Can you work these out from the drawing? Everything is in mm from the part's minimum corner. Coordinates: 2 decimals unless noted, no trailing zeros. Order: outer loops, then holes, each group sorted by start corner. A loop starts at its lowest first (then second) coordinate and runs counter-clockwise, first axis right, second up. Notation, with made-up numbers: (47, 2) - (89, 2) arc R7 cw to (89, 11) - close; hole circle Ø1 at (-25.75, 88.25). An arc over 180 degrees is marked (long way). Use a Markdown table: item, result. Add a question column.
(1) I want a section at C-C (y = 1.5). List the corners of the cut face in (x, z) for me.
(2) I want a section at A-A (y = 4.75). List the corners of the cut face in (x, z) for me (1 decimal).
(3) I want a section at B-B (z = 1). List the corners of the cut face in (x, y) for me (1 decimal).
(4) If I drill on L1, parallel to X at y = 1.25, z = 0.5; L2, parallel to X at y = 6.75, z = 0.35 (1 decimal); L3, parallel to Y at x = 19, z = 0.2 (1 decimal), over which ranges is the centre line in solid material (lowest first)? Write a range as [from, to].
(5) We'd pull the mould along X, two halves only. Please class the marked faces 1 and 2: pulls with the +X half, pulls with the -X half, needs draft (parallel to the pull), parting line crosses it, or undercut.
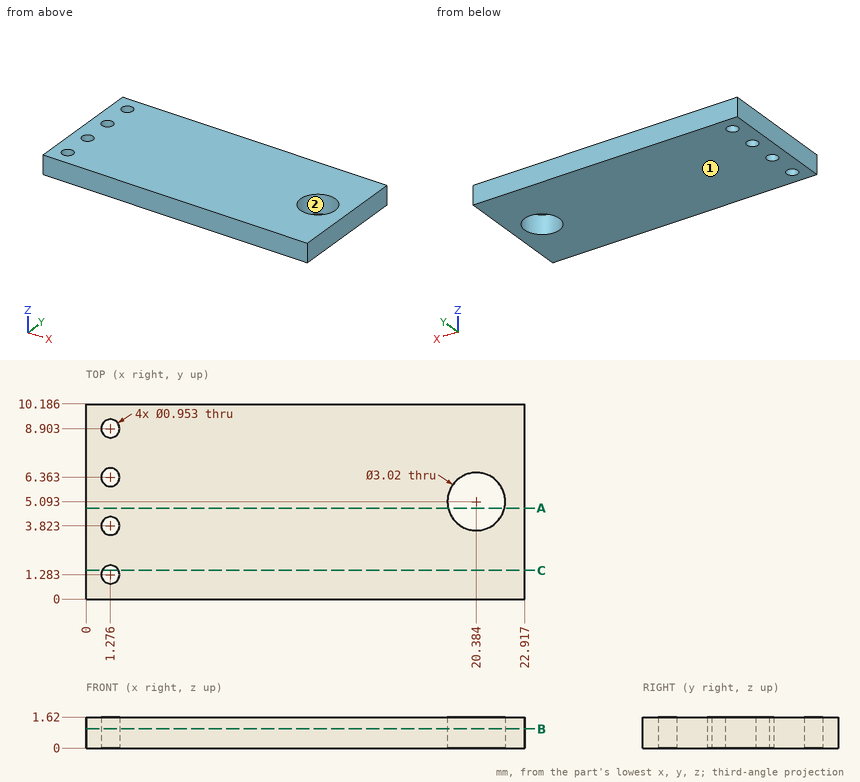
Answers follow:
| question | item | result |
|---|---|---|
| 1 | outline | (0, 0) - (0.85, 0) - (0.85, 1.62) - (0, 1.62) - close; (1.7, 0) - (22.92, 0) - (22.92, 1.62) - (1.7, 1.62) - close |
| 2 | outline | (0, 0) - (18.9, 0) - (18.9, 1.6) - (0, 1.6) - close; (21.9, 0) - (22.9, 0) - (22.9, 1.6) - (21.9, 1.6) - close |
| 3 | outline | (0, 0) - (22.9, 0) - (22.9, 10.2) - (0, 10.2) - close; hole circle Ø1 at (1.3, 1.3); hole circle Ø1 at (1.3, 3.8); hole circle Ø1 at (1.3, 6.4); hole circle Ø1 at (1.3, 8.9); hole circle Ø3 at (20.4, 5.1) |
| 4 | L1 | x = [0, 0.8], [1.75, 22.92] |
| 4 | L2 | x = [0, 1], [1.6, 22.9] |
| 4 | L3 | y = [0, 4.5], [5.7, 10.2] |
| 5 | face 1 | needs draft |
| 5 | face 2 | undercut |
